from build123d import *

# Parameters (mm, degrees)
SKETCH1_W           = 2.54
SKETCH1_H           = 2.54
SKETCH1_W_2         = 1.14
SKETCH1_H_2         = 1.14
BOSS_EXTRUDE1_DEPTH = 12
SKETCH2_W           = 2.04
SKETCH2_H           = 2.04
CUT_EXTRUDE1_DEPTH  = 11.5
CHAMFER1_SIZE       = 0.3
SKETCH3_W           = 2.54
SKETCH3_H           = 5
CUT_EXTRUDE2_DEPTH  = 0.25
BOSS_EXTRUDE2_DEPTH = 0.9


with BuildPart() as part:
    # Sketch1 → Boss-Extrude1 (new body)
    with BuildSketch(Plane.XY):
        Rectangle(SKETCH1_W, SKETCH1_H)
        Rectangle(SKETCH1_W_2, SKETCH1_H_2, mode=Mode.SUBTRACT)
    extrude(amount=BOSS_EXTRUDE1_DEPTH)

    # Sketch2 → Cut-Extrude1 (cut)
    with BuildSketch(Plane.XY.offset(12)):
        Rectangle(SKETCH2_W, SKETCH2_H)
    extrude(amount=-CUT_EXTRUDE1_DEPTH, mode=Mode.SUBTRACT)

    # Chamfer1
    chamfer1_edges = [part.edges().sort_by_distance(p)[0] for p in [
        (0.57, 0, 0),
        (0, 0.57, 0),
        (-0.57, 0, 0),
        (0, -0.57, 0),
    ]]
    chamfer(chamfer1_edges, length=CHAMFER1_SIZE)

    # Sketch3 → Cut-Extrude2 (cut)
    with BuildSketch(Plane.XZ.offset(1.27)):
        with Locations((0, 6.2)):
            Rectangle(SKETCH3_W, SKETCH3_H)
    extrude(amount=-CUT_EXTRUDE2_DEPTH, mode=Mode.SUBTRACT)

    # Sketch4 → Boss-Extrude2 (add, symmetric)
    with BuildSketch(Plane(origin=(0, 0, 0), x_dir=(0, 0, -1), z_dir=(1, 0, 0))):
        Polygon((-5.3, -1.51689304), (-5.3, -0.798560217), (-8.7, -1.02), (-8.7, -1.27), align=None)
    extrude(amount=BOSS_EXTRUDE2_DEPTH, both=True)


solid = part.part
Geometry: final body of the model. Coordinates: model frame, mm. A direction names the side the tool comes from. Round coordinates to 2 decimals unless told otherwise and drop trailing zeros. Order: outer loops, then holes, each group sorted by start corner. A loop starts at its lowest first (then second) coordinate and runs counter-clockwise, first axis right, second up. Notation, with made-up numbers: (55, 35.25) -> (114, 35.25) arc R25 cw to (114, 49.25) -> close; hole circle Ø2 at (29.25, 46.25). An arc over 180 degrees is marked (long way). Put each result on its own line as item: value. Start each with the question number.
Q1. Section C-C on y = -0.4. Return the cut outline in (x, z), and give its area (3 significant figures).
Q2. Section B-B on x = 0.7. Return the cut outline in (y, z).
Q3. First-contact query: pin 1 (1.5 mm diameter, centred on x = 0.5, z = 7.5, fed in from -Y); pin 2 (0.8 mm diameter, centred on y = -1.5, z = 7, fed in from -X); pin 3 (0.8 mm diameter, centred on y = -1.5, z = 6.5, fed in from +X). Flat tips, straight axial feed; report the tip coordinate or a pass-through.
Q4. Pull-direction query (X, two-part tool) for faces 4 (the flat face through (0, -1.02, 2)), 5 (the flat face through (1.27, 0, 6)), 6 (the flat face through (1.02, 0, 6)), 7 (the flat face through (0, -1.27, 2)); classes: +X half, -X half, draft (parallel to the pull), parting line (faces both ways), or undercut.
Q5. Section A-A on x = 0.15. Return the cut outline in (y, z).
Q6. Line query: probe 1 along Y at (x, z) = (-0.35, 11); probe 2 along Z at (x, y) = (1.15, -1.1). Output: solid intervals per line, ascending.
Q7. Section D-D on z = 9.25. Return the cut outline in (x, y).
Q8. Reachability of faces 1 (the flat face through (0, -1.02, 10)), 2 (the flat face through (0, -1.27, 10)), 3 (the flat face through (0, 1.27, 6)) from +Z, -Z, +X, -X, +Y, -Y: full face, straight path, thin tool, end or side. Return the list, or none.
Ans:
1. outline: (-1.27, 0) -> (-0.87, 0) -> (-0.57, 0.3) -> (-0.57, 0.5) -> (-1.02, 0.5) -> (-1.02, 12) -> (-1.27, 12) -> close; (0.57, 0.3) -> (0.87, 0) -> (1.27, 0) -> (1.27, 12) -> (1.02, 12) -> (1.02, 0.5) -> (0.57, 0.5) -> close
1. area: 6.36 mm2
2. outline: (-1.52, 5.3) -> (-0.8, 5.3) -> (-1.02, 8.7) -> (-1.02, 12) -> (-1.27, 12) -> (-1.27, 8.7) -> close; (-1.27, 0) -> (-0.87, 0) -> (-0.7, 0.17) -> (0.7, 0.17) -> (0.87, 0) -> (1.27, 0) -> (1.27, 12) -> (1.02, 12) -> (1.02, 0.5) -> (-1.02, 0.5) -> (-1.02, 3.7) -> (-1.27, 3.7) -> close
3. pin 1: stops at y = -1.41
3. pin 2: stops at x = -0.9
3. pin 3: stops at x = 0.9
4. face 4: undercut
4. face 5: +X half
4. face 6: undercut
4. face 7: draft
5. outline: (-1.52, 5.3) -> (-0.8, 5.3) -> (-1.02, 8.7) -> (-1.02, 12) -> (-1.27, 12) -> (-1.27, 8.7) -> close; (-1.27, 0) -> (-0.87, 0) -> (-0.57, 0.3) -> (-0.57, 0.5) -> (-1.02, 0.5) -> (-1.02, 3.7) -> (-1.27, 3.7) -> close; (0.57, 0.3) -> (0.87, 0) -> (1.27, 0) -> (1.27, 12) -> (1.02, 12) -> (1.02, 0.5) -> (0.57, 0.5) -> close
6. probe 1: y = -1.27 to -1.02, 1.02 to 1.27
6. probe 2: z = 0 to 3.7, 8.7 to 12
7. outline: (-1.27, -1.27) -> (1.27, -1.27) -> (1.27, 1.27) -> (-1.27, 1.27) -> close; hole (-1.02, -1.02) -> (1.02, -1.02) -> (1.02, 1.02) -> (-1.02, 1.02) -> close
8. face 1: +Z
8. face 2: +Z, +X, -X, -Y
8. face 3: +Z, -Z, +X, -X, +Y
